from build123d import *

# Parameters (mm, degrees)
F0_W         = 152.4
F0_H         = 19.05
F1_DEPTH     = 1.5875
F2_SIZE      = 9.52499
F3_W         = 9.525
F3_H         = 5.08
F4_DEPTH     = 4.7625
F5_SIZE      = 1.27
F6_W         = 5.08
F6_H         = 0.762
F7_DEPTH     = 1.27
F8_SIZE      = 1.524
F9_T1_DEPTH  = 19.1535983177
F9_T3_DEPTH  = 7.8385097473
F9_T5_DEPTH  = 21.3088597868
F9_T7_DEPTH  = 150.7134997473
F9_T9_DEPTH  = 25.3644897473
F9_T14_DEPTH = 9.4899593576
F9_T19_DEPTH = 9.4899593576
F9_T24_DEPTH = 9.4899593576
F9_T29_DEPTH = 9.4899593576


# Not quite as in the source:
# - a fillet or chamfer that OpenCascade refuses, or shapes differently, is made with other operations: its cross-section is extruded or revolved along the edge and cut away or added
# - two fillets or chamfers of one size are made in one step
# - a fillet or chamfer is up to 0.001 mm smaller than in the source, because OpenCascade refuses the exact size


with BuildPart() as f1:
    # F0 (on Top) → F1 (new body)
    with BuildSketch(Plane.XY):
        with Locations((2.4961568415, 22.6473969003)):
            Rectangle(F0_W, F0_H)
    extrude(amount=-F1_DEPTH)

    # F2 (size 9.525 in the source; OpenCascade refuses exactly that, so slightly less here)
    f2_edges = [f1.edges().sort_by_distance(p)[0] for p in [
        (78.696157, 13.122397, -0.79375),
        (78.696157, 32.172397, -0.79375),
    ]]
    chamfer(f2_edges, length=F2_SIZE)

    # F3 (on face) → F4 (join)
    with BuildSketch(Plane.XY):
        with Locations((-48.8753431585, 22.6473969003)):
            Rectangle(F3_W, F3_H)
    extrude(amount=F4_DEPTH)

    # F5
    f5_edges = [f1.edges().sort_by_distance(p)[0] for p in [
        (-44.112843, 20.107397, 2.38125),
        (-44.112843, 25.187397, 2.38125),
        (-48.875343, 25.187397, 4.7625),
        (-48.875343, 20.107397, 4.7625),
    ]]
    chamfer(f5_edges, length=F5_SIZE)

    # F6 (on face) → F7 (cut)
    with BuildSketch(Plane(origin=(-53.6378431585, 0, 0), x_dir=(0, -1, 0), z_dir=(-1, 0, 0))):
        with Locations((-22.6473969003, 3.1115)):
            Rectangle(F6_W, F6_H)
    extrude(amount=-F7_DEPTH, mode=Mode.SUBTRACT)

    # F8
    f8_edges = [f1.edges().sort_by_distance(p)[0] for p in [
        (-2.266338, 13.122397, 0),
    ]]
    chamfer(f8_edges, length=F8_SIZE)

    # F9: chamfer of 1.524 on 7 edges, made by hand

    # F9_s2 → F9_t1 (cut)
    with BuildSketch(Plane(origin=(53.4430964982, 53.4430964982, 0), x_dir=(0, 0, 1), z_dir=(-0.7071067812, -0.7071067812, 0))):
        Polygon((0, -38.1084653026), (-1.524, -39.6324653026), (0, -39.6324653026), align=None)
    extrude(amount=F9_T1_DEPTH, mode=Mode.SUBTRACT)

    # F9_s4 → F9_t3 (cut)
    with BuildSketch(Plane.XZ.offset(-26.566651774)):
        Polygon((77.1721568415, 0), (78.6961568415, -1.524), (78.6961568415, 0), align=None)
    extrude(amount=F9_T3_DEPTH, mode=Mode.SUBTRACT)

    # F9_s6 → F9_t5 (cut)
    with BuildSketch(Plane(origin=(30.7956995979, -30.7956995979, 0), x_dir=(0, 0, 1), z_dir=(-0.7071067812, 0.7071067812, 0))):
        Polygon((0, 70.1367211515), (-1.524, 71.6607211515), (0, 71.6607211515), align=None)
    extrude(amount=F9_T5_DEPTH, mode=Mode.SUBTRACT)

    # F9_s8 → F9_t7 (cut)
    with BuildSketch(Plane.YZ.offset(-77.6230880321)):
        Polygon((30.6483969003, 0), (32.1723969003, -1.524), (32.1723969003, 0), align=None)
    extrude(amount=F9_T7_DEPTH, mode=Mode.SUBTRACT)

    # F9_s10 → F9_t9 (cut)
    with BuildSketch(Plane.XZ.offset(-36.091641774)):
        Polygon((-72.1798431585, 0), (-73.7038431585, -1.524), (-73.7038431585, 0), align=None)
    extrude(amount=F9_T9_DEPTH, mode=Mode.SUBTRACT)


with BuildPart() as f9_tool12:
    # F9_s13 → F9_t14 (new body)
    with BuildSketch(Plane.XY.offset(3.9512296788)):
        Polygon((77.618526107, 21.5697561658), (78.6961568415, 24.1713869003), (78.6961568415, 22.6473869003), align=None)
    extrude(amount=-F9_T14_DEPTH)

    split(bisect_by=Plane(origin=(38.5860784208, 0, 38.5860784208), x_dir=(0, 1, 0), z_dir=(0.7071067812, 0, 0.7071067812)), keep=Keep.TOP)


with BuildPart() as f1_1:
    add(f1.part)

    # F9_t11: cut F9_tool12
    add(f9_tool12.part, mode=Mode.SUBTRACT)


with BuildPart() as f9_tool17:
    # F9_s18 → F9_t19 (new body)
    with BuildSketch(Plane.XY.offset(3.9512296788)):
        Polygon((77.618526107, 21.5697561658), (78.6961568415, 24.1713869003), (78.6961568415, 22.6473869003), align=None)
    extrude(amount=-F9_T19_DEPTH)

    split(bisect_by=Plane(origin=(13.473377118, -13.473377118, 19.0542326513), x_dir=(0.7071067812, 0.7071067812, 0), z_dir=(0.5, -0.5, 0.7071067812)), keep=Keep.TOP)


with BuildPart() as f1_2:
    add(f1_1.part)

    # F9_t16: cut F9_tool17
    add(f9_tool17.part, mode=Mode.SUBTRACT)


with BuildPart() as f9_tool22:
    # F9_s23 → F9_t24 (new body)
    with BuildSketch(Plane.XY.offset(3.9512296788)):
        Polygon((78.6961568415, 21.1234069003), (77.618526107, 23.7250376349), (78.6961568415, 22.6474069003), align=None)
    extrude(amount=-F9_T24_DEPTH)

    split(bisect_by=Plane(origin=(24.7970755682, 24.7970755682, 35.0683605757), x_dir=(-0.7071067812, 0.7071067812, 0), z_dir=(0.5, 0.5, 0.7071067812)), keep=Keep.TOP)


with BuildPart() as f1_3:
    add(f1_2.part)

    # F9_t21: cut F9_tool22
    add(f9_tool22.part, mode=Mode.SUBTRACT)


with BuildPart() as f9_tool27:
    # F9_s28 → F9_t29 (new body)
    with BuildSketch(Plane.XY.offset(3.9512296788)):
        Polygon((78.6961568415, 21.1234069003), (77.618526107, 23.7250376349), (78.6961568415, 22.6474069003), align=None)
    extrude(amount=-F9_T29_DEPTH)

    split(bisect_by=Plane(origin=(38.5860784208, 0, 38.5860784208), x_dir=(0, 1, 0), z_dir=(0.7071067812, 0, 0.7071067812)), keep=Keep.TOP)


with BuildPart() as f1_4:
    add(f1_3.part)

    # F9_t26: cut F9_tool27
    add(f9_tool27.part, mode=Mode.SUBTRACT)


solid = f1_4.part
Input: part model. Units: mm. Frame: model coordinates. A direction names the side the tool comes from. Round coordinates to 2 decimals unless told otherwise and drop trailing zeros. Order: outer loops, then holes, each group sorted by start corner. A loop starts at its lowest first (then second) coordinate and runs counter-clockwise, first axis right, second up. Notation, with made-up numbers: (-9.75, 6.25) - (28.25, 6.25) arc R22 cw to (28.25, 37.25) - close; hole circle Ø8 at (-26, 35). An arc over 180 degrees is marked (long way). Answer as a JSON object with one key per item and string values. Group by question number.
(1) Reachability of faces 1 (the face through (-44.113, 23, 2)), 2 (the face through (-53.638, 23, 1)), 3 (the face through (-50, 25.187, 2)) from +Z, -Z, +X, -X, +Y, -Y: full face, straight path, thin tool, end or side. Return the list, or none.
(2) Cut plane B-B (y = 29). Return loops of the section in (x, z), then the cut area to 3 significant figures.
(3) Cut plane A-A (x = 6). Return loops of the section in (y, z), then the cut area to 3 significant figures.
(4) Material intervals for probe 1 along Z at (x, y) = (-60, 28.25); probe 2 along X at (y, z) = (23.75, 4); probe 3 along X at (y, z) = (20.75, -0.5), sorted ascending. Write a range as from..to.
(5) Pin query (flat end, axial travel): P1, Ø4, axis at x = 15.5, y = 16, coming from the +Z side; P2, Ø3, axis at x = -49, z = 2.5, coming from the -Y side; P3, Ø0.8, axis at y = 22.5, z = 2.5, coming from the +X side. Return the tip coordinate at first contact, or that it passes through.
Here are the results:
{
 "1": {"face 1": "+Z, +X, +Y, -Y", "face 2": "+Z, -X, +Y, -Y", "face 3": "+Z, +X, -X, +Y"},
 "2": {"outline": "(-73.7, -1.59) - (72.34, -1.59) - (72.34, -1.52) - (70.19, 0) - (-72.18, 0) - (-73.7, -1.52) - close", "area": "229 mm^2"},
 "3": {"outline": "(13.12, -1.59) - (32.17, -1.59) - (32.17, -1.52) - (30.65, 0) - (14.65, 0) - (13.12, -1.52) - close", "area": "27.9 mm^2"},
 "4": {"probe 1": "z = -1.59..0", "probe 2": "x = -53.64..-44.11", "probe 3": "x = -72.68..75.35"},
 "5": {"P1": "stops at z = 0", "P2": "stops at y = 20.11", "P3": "stops at x = -44.11"}
}
